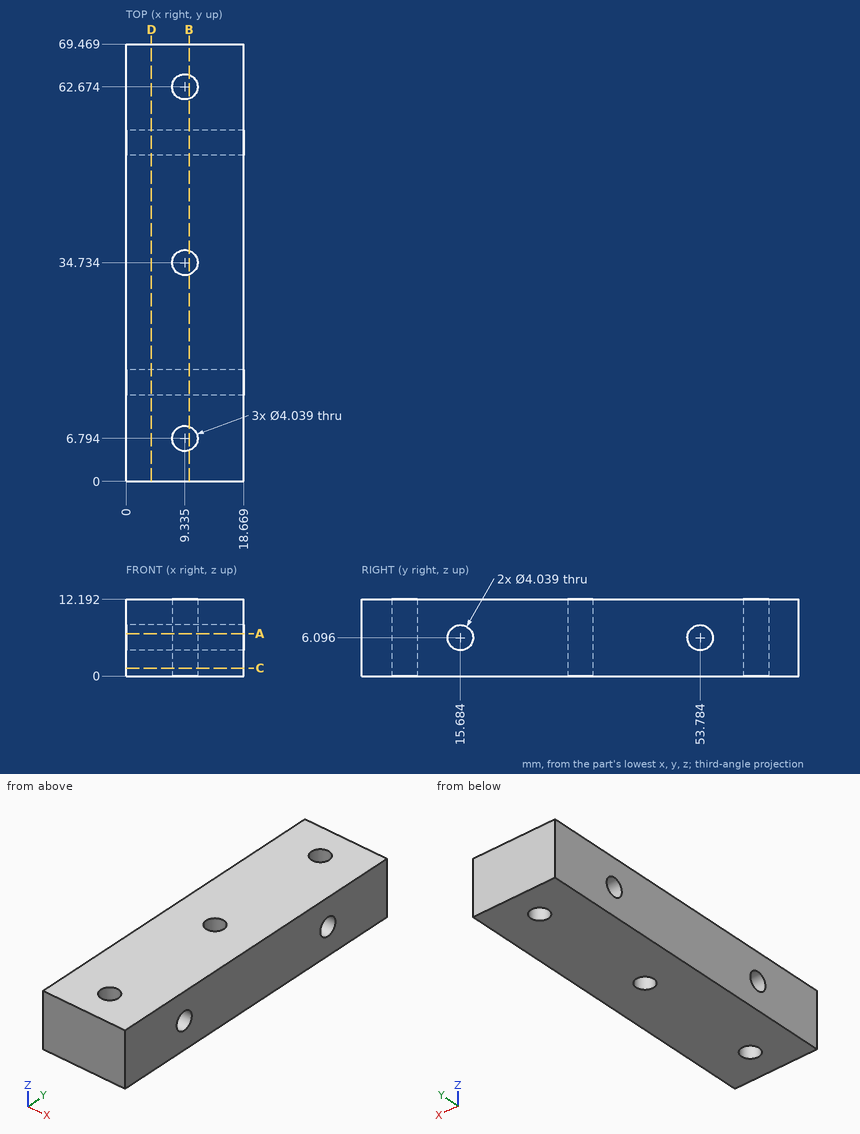
Drawing for the job (mm, zero at the part's lowest x, y, z). Give positions to 0.01 mm unless a question says otherwise; leave off trailing zeros. Order: outer loops, then holes, each group sorted by start corner. A loop starts at its lowest first (then second) coordinate and runs counter-clockwise, first axis right, second up. Notation, with made-up numbers: M 35,16 L 48,16 A23 cw 48,49 Z; hole C 87,6.5 d1. An arc over 180 degrees is marked long. Write item = value, one per line. Start each with the question number.
(1) Slice it at D-D on x = 4. Write the cut outline in (y, z) (1 decimal).
(2) Slice it at A-A on z = 6.75. Write the cut outline in (x, y) (1 decimal).
(3) Slice it at B-B on x = 10. Write the cut outline in (y, z) (1 decimal).
(4) Pin check, flat tips, straight feed: pin 1 Ø3 at (y, z) = (15.68, 6.1) entering from +X; pin 2 Ø5.5 at (y, z) = (53.78, 6.1) entering from -X. Stop position of each tip, or through.
(5) Probe L1, parallel to Y at x = 16.5, z = 6.25; L2, parallel to Y at x = 9.5, z = 10.25; L3, parallel to Y at x = 10.5, z = 1.75 (1 decimal). List the from-to ranges inside material, lowest first. Write a range as [from, to].
(6) Slice it at C-C on z = 1.25. Write the cut outline in (x, y) (1 decimal).
Responses:
q1.outline = M 0,0 L 69.5,0 L 69.5,12.2 L 0,12.2 Z; hole C 15.7,6.1 d4; hole C 53.8,6.1 d4
q2.outline = M 0,0 L 18.7,0 L 18.7,13.8 L 0,13.8 Z; M 0,17.6 L 18.7,17.6 L 18.7,51.9 L 0,51.9 Z; M 0,55.7 L 18.7,55.7 L 18.7,69.5 L 0,69.5 Z; hole C 9.3,6.8 d4; hole C 9.3,34.7 d4; hole C 9.3,62.7 d4
q3.outline = M 0,0 L 4.9,0 L 4.9,12.2 L 0,12.2 Z; M 8.7,0 L 32.8,0 L 32.8,12.2 L 8.7,12.2 Z; M 36.6,0 L 60.8,0 L 60.8,12.2 L 36.6,12.2 Z; M 64.6,0 L 69.5,0 L 69.5,12.2 L 64.6,12.2 Z; hole C 15.7,6.1 d4; hole C 53.8,6.1 d4
q4.pin_1 = through
q4.pin_2 = 0
q5.L1 = [0, 13.67], [17.7, 51.77], [55.8, 69.47]
q5.L2 = [0, 4.78], [8.81, 32.72], [36.75, 60.66], [64.69, 69.47]
q5.L3 = [0, 5.1], [8.4, 33.1], [36.4, 61], [64.3, 69.5]
q6.outline = M 0,0 L 18.7,0 L 18.7,69.5 L 0,69.5 Z; hole C 9.3,6.8 d4; hole C 9.3,34.7 d4; hole C 9.3,62.7 d4
